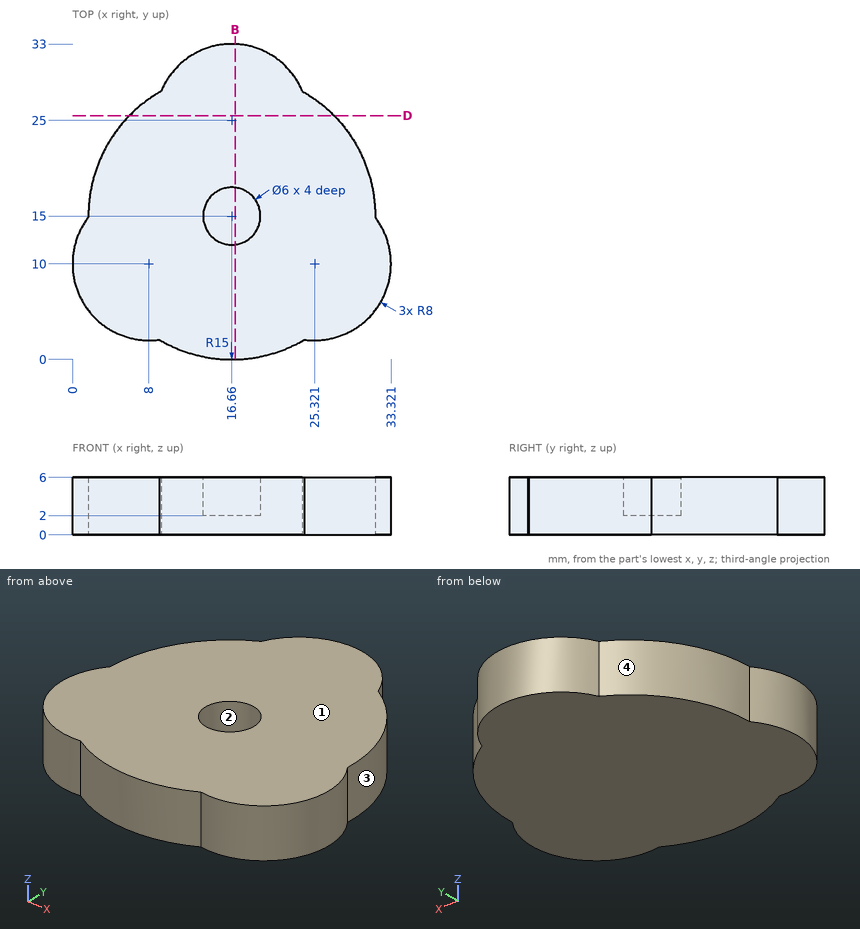
Source: three-view drawing plus pictorial views. Frame: mm from the lowest corner of the part. Round coordinates to 2 decimals unless told otherwise and drop trailing zeros. Loops run counter-clockwise (first coordinate to the right, second up) from the corner with the lowest first, then second, coordinate; pieces in that order, holes last.
Q1. Section D-D, the plane y = 25.5. Return loops of the section in (x, z).
Q2. First-contact query: P1, Ø1.8, axis at x = 17, y = 15.5, coming from the +Z side; P2, Ø3, axis at x = 20.5, z = 3, coming from the -Y side. Flat tips, straight axial feed; report the tip coordinate or a pass-through.
Q3. Mould query, pull axis X, two halves, no side actions, for the marked faces 1, 2, 3 and 4. Classes: pulls with the +X half, pulls with the -X half, needs draft (parallel to the pull), parting line crosses it, or undercut.
Q4. Ray query, line 1 (Y direction, x = 18, z = 5.15) (1 decimal); line 2 (Y direction, x = 14, z = 2.9) (1 decimal); line 3 (X direction, y = 21.5, z = 1.45). Return the intervals inside material, ascending.
Q5. Section B-B, the plane x = 17. Return loops of the section in (y, z).
Solutions:
1. outline: (5.95, 0) - (27.37, 0) - (27.37, 6) - (5.95, 6) - close
2. P1: stops at z = 2
2. P2: stops at y = 0.18
3. face 1: needs draft
3. face 2: undercut
3. face 3: pulls with the +X half
3. face 4: pulls with the -X half
4. line 1: y = 0.1 to 12.3, 17.7 to 32.9
4. line 2: y = 0.2 to 13.6, 16.4 to 32.5
4. line 3: x = 3.14 to 30.18
5. outline: (0, 0) - (32.99, 0) - (32.99, 6) - (17.98, 6) - (17.98, 2) - (12.02, 2) - (12.02, 6) - (0, 6) - close
